```python
from build123d import *

# Parameters (mm, degrees)
F0_W     = 1600
F0_H     = 1980
F1_DEPTH = 380
F2_DEPTH = 1000
F3_DEPTH = 5


with BuildPart() as f1:
    # F0 (on Top) → F1 (new body)
    with BuildSketch(Plane.XY):
        Polygon((-800, 1000), (-880, 1000), (-880, -1045), (880, -1045), (880, 1000), (800, 1000), align=None)
        with Locations((0, -10)):
            Rectangle(F0_W, F0_H, mode=Mode.SUBTRACT)
    extrude(amount=F1_DEPTH)

    # F0 (on Top) → F2 (join)
    with BuildSketch(Plane.XY):
        Polygon((880, 1045), (-880, 1045), (-880, 1000), (-800, 1000), (800, 1000), (880, 1000), align=None)
    extrude(amount=F2_DEPTH)

    # F0 (on Top) → F3 (join)
    with BuildSketch(Plane.XY):
        with Locations((0, -10)):
            Rectangle(F0_W, F0_H)
    extrude(amount=F3_DEPTH)


solid = f1.part
```
Can you work these out from the model? Positions are in its coordinate system, mm. A direction names the side the tool comes from. Coordinates: 2 decimals unless noted, no trailing zeros. Order: outer loops, then holes, each group sorted by start corner. A loop starts at its lowest first (then second) coordinate and runs counter-clockwise, first axis right, second up.
1. If we section it at B-B (z = 277.5): Please give me the cut outline in (x, y).
2. I'm going to push flat-ended pins straight in: pin 1 (2 mm diameter, centred on x = 612.5, z = 715.5, fed in from -Y); pin 2 (4 mm diameter, centred on x = 95.5, y = -736.5, fed in from +Z). Where does each tip first touch, or does it pass through?
3. If we section it at C-C (y = 741): Please give me the cut outline in (x, z).
4. If we section it at D-D (z = 613): Please give me the cut outline in (x, y), then the cut area to 3 significant figures.
5. I need wall thicknesses on line 1 (X direction, y = 780, z = 230.5); line 2 (Y direction, x = -526, z = 241); line 3 (Y direction, x = -33.5, z = 935). Which ranges of each line are inside material? Lowest first, please.
6. If we section it at A-A (x = 603.5): Please give me the cut outline in (y, z).
7. Thinking about a two-plate mould opening in X: for faces 1 (the face through (-12, -1045, 187)), 2 (the face through (880, 73, 201)), 3 (the face through (-11, -1000, 190)), which applies, +X half, -X half, draft (parallel to the pull), parting line (faces both ways), or undercut?
8. For faces 4 (the face through (-12, 1000, 686)), 5 (the face through (-12, 1023, 1000)), 6 (the face through (-11, 980, 190)), which set-ups out of +Z, -Z, +X, -X, +Y, -Y let a thin tool reach every point of the face, with its end or its side?
Entries:
1. outline: (-880, -1045) - (880, -1045) - (880, 1045) - (-880, 1045) - close; hole (-800, -1000) - (800, -1000) - (800, 980) - (-800, 980) - close
2. pin 1: stops at y = 1000
2. pin 2: stops at z = 5
3. outline: (-880, 0) - (880, 0) - (880, 380) - (800, 380) - (800, 5) - (-800, 5) - (-800, 380) - (-880, 380) - close
4. outline: (-880, 1000) - (880, 1000) - (880, 1045) - (-880, 1045) - close
4. area: 79,200 mm2
5. line 1: x = -880 to -800, 800 to 880
5. line 2: y = -1045 to -1000, 980 to 1045
5. line 3: y = 1000 to 1045
6. outline: (-1045, 0) - (1045, 0) - (1045, 1000) - (1000, 1000) - (1000, 380) - (980, 380) - (980, 5) - (-1000, 5) - (-1000, 380) - (-1045, 380) - close
7. face 1: draft
7. face 2: +X half
7. face 3: undercut
8. face 4: +Z, +X, -X, -Y
8. face 5: +Z, +X, -X, +Y, -Y
8. face 6: +Z
